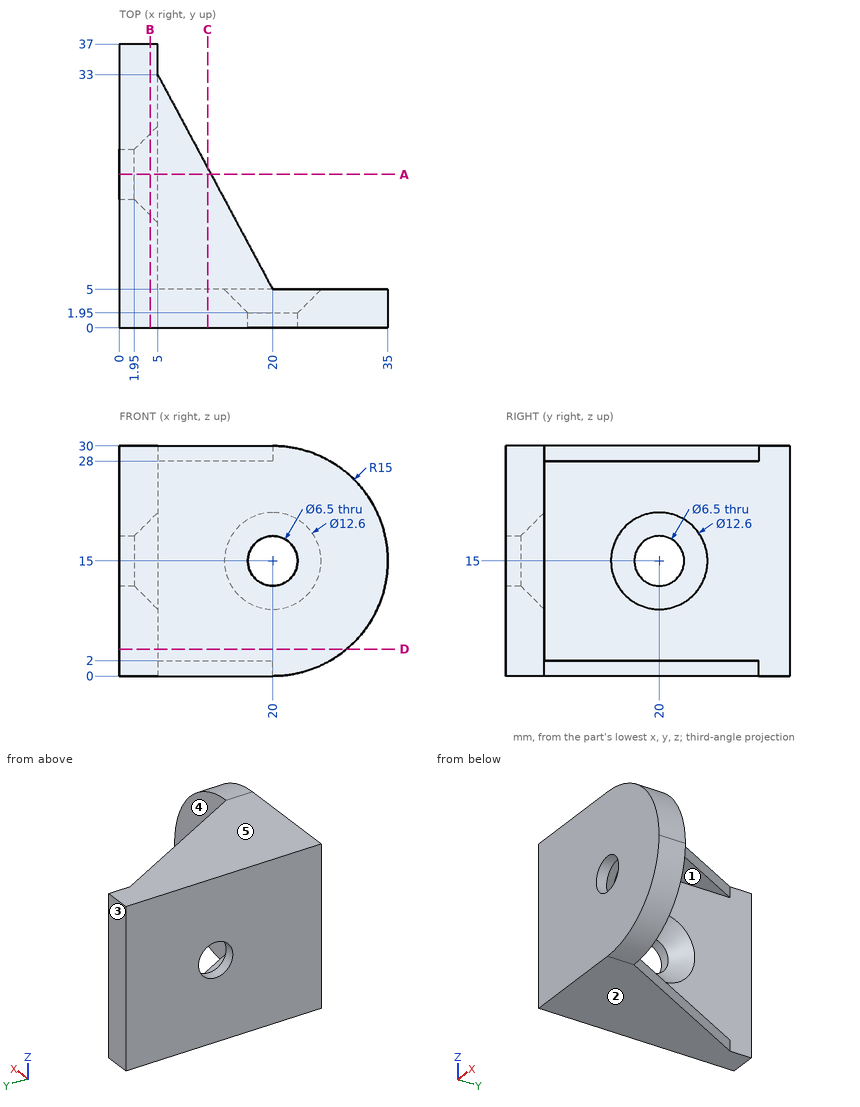
Print and shaded views of the part. All mm, measured from the part's lowest x, y and z. A direction names the side the tool comes from. Give positions to 0.01 mm unless a question says otherwise; leave off trailing zeros. Loops run counter-clockwise (first coordinate to the right, second up) from the corner with the lowest first, then second, coordinate; pieces in that order, holes last. Notation, with made-up numbers: (-1, -28.5) -> (25, -28.5) arc R17 ccw to (25, -7.5) -> close; hole circle Ø7 at (4, -17). An arc over 180 degrees is marked (long way). Use CSV: the item, a comma, the result in double quotes. Start each with the question number.
1) Slice it at C-C on x = 11.5. Give the cut face in (y, z).
2) Flat gauge pins, fed straight in: pin 1 Ø1.5 at (y, z) = (26.5, 24.5) entering from +X; pin 2 Ø5 at (x, y) = (26, 8) entering from +Z; pin 3 Ø10.5 at (x, z) = (20, 15) entering from -Y; pin 4 Ø8 at (x, y) = (29.5, 4.5) entering from +Z. Where does each tip first touch, or does it go through?
3) Slice it at A-A on y = 20. Give the cut face in (x, z).
4) Mould opens along Z. For the marked faces 3, 4 and 5 say: released by +Z, released by -Z, zero draft, split by the parting line, or undercut.
5) Tool access for the marked faces 1 and 2: list every direction of +Z, -Z, +X, -X, +Y, -Y with a clear straight run to the whole face (end or side of a thin tool).
6) Slice it at B-B on x = 4. Give the cut face in (y, z), plus the area to 3 significant figures.
7) Slice it at D-D on z = 3.5. Give the cut face in (x, y), plus the area to 3 significant figures.
8) Wall check: line 1 (Z direction, x = 20, y = 0.75); line 2 (Z direction, x = 6, y = 21); line 3 (X direction, y = 1.1, z = 15). Give the ranges that are in metal, low to high.
Computed values:
1,outline,"(0, 0) -> (20.87, 0) -> (20.87, 2) -> (5, 2) -> (5, 28) -> (20.87, 28) -> (20.87, 30) -> (0, 30) -> close"
2,pin 1,"stops at x = 5"
2,pin 2,"passes through"
2,pin 3,"stops at y = 0"
2,pin 4,"stops at z = 28.96"
3,outline,"(0, 0) -> (11.96, 0) -> (11.96, 2) -> (5, 2) -> (5, 8.7) -> (1.95, 11.75) -> (0, 11.75) -> close; (0, 18.25) -> (1.95, 18.25) -> (5, 21.3) -> (5, 28) -> (11.96, 28) -> (11.96, 30) -> (0, 30) -> close"
4,face 3,"zero draft"
4,face 4,"undercut"
4,face 5,"released by +Z"
5,face 1,"+X, +Y"
5,face 2,"-Z, +X, -X, +Y, -Y"
6,outline,"(0, 0) -> (37, 0) -> (37, 30) -> (0, 30) -> close; hole circle Ø10.6 at (20, 15)"
6,area,"1,020 mm^2"
7,outline,"(0, 0) -> (29.63, 0) -> (29.63, 5) -> (5, 5) -> (5, 37) -> (0, 37) -> close"
7,area,"308 mm^2"
8,line 1,"z = 0 to 11.75, 18.25 to 30"
8,line 2,"z = 0 to 2, 28 to 30"
8,line 3,"x = 0 to 16.75, 23.25 to 35"
